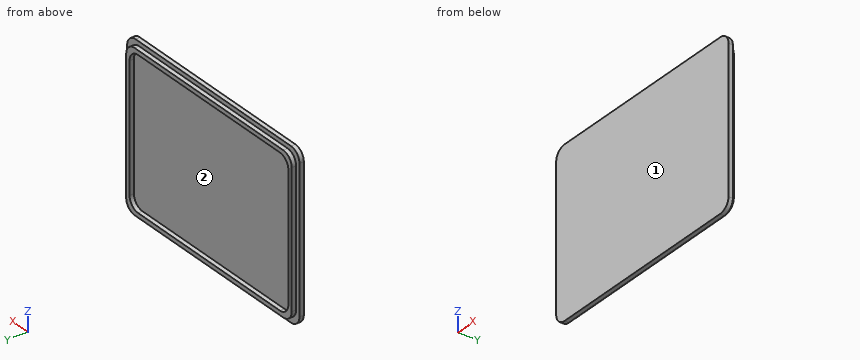
```python
from build123d import *

# Parameters (mm, degrees)
SKETCH1_W           = 101.6
SKETCH1_H           = 76.2
BOSS_EXTRUDE1_DEPTH = 2
SKETCH2_W           = 97.6
SKETCH2_H           = 72.2
SKETCH2_W_2         = 93.6
SKETCH2_H_2         = 68.2
EXTRUDE_THIN1_DEPTH = 2
FILLET1_R           = 5
FILLET2_R           = 5


with BuildPart() as part:
    # Sketch1 → Boss-Extrude1 (new body)
    with BuildSketch(Plane(origin=(0, 0, 0), x_dir=(1, 0, 0), z_dir=(0, 1, 0))):
        Rectangle(SKETCH1_W, SKETCH1_H)
    extrude(amount=BOSS_EXTRUDE1_DEPTH)

    # Sketch2 → Extrude-Thin1 (add)
    with BuildSketch(Plane(origin=(0, 2, 0), x_dir=(1, 0, 0), z_dir=(0, 1, 0))):
        Rectangle(SKETCH2_W, SKETCH2_H)
        Rectangle(SKETCH2_W_2, SKETCH2_H_2, mode=Mode.SUBTRACT)
    extrude(amount=EXTRUDE_THIN1_DEPTH)

    # Fillet1
    fillet1_edges = [part.edges().sort_by_distance(p)[0] for p in [
        (50.8, 1, 38.1),
        (-50.8, 1, 38.1),
        (-50.8, 1, -38.1),
        (50.8, 1, -38.1),
    ]]
    fillet(fillet1_edges, radius=FILLET1_R)

    # Fillet2
    fillet2_edges = [part.edges().sort_by_distance(p)[0] for p in [
        (48.8, 3, -36.1),
        (-48.8, 3, -36.1),
        (-48.8, 3, 36.1),
        (48.8, 3, 36.1),
        (-46.8, 3, -34.1),
        (-46.8, 3, 34.1),
        (46.8, 3, 34.1),
        (46.8, 3, -34.1),
    ]]
    fillet(fillet2_edges, radius=FILLET2_R)


solid = part.part
```
Verification items for the finished model (mm, model axes). Face numbers are marked on the shaded views. Round coordinates to 2 decimals unless told otherwise and drop trailing zeros. Write each loop counter-clockwise with the first axis right and the second up, starting at its lowest first coordinate (ties: lowest second). Pieces come first, ordered by that corner, then holes. Notation, with made-up numbers: (86, 7.5) - (126, 7.5) arc R17 cw to (126, 33.5) - close; hole circle Ø10 at (85, 84). An arc over 180 degrees is marked (long way). Answer as a JSON object with one key per item and string values. Group by question number.
Q1. Go/stop test with flat-tipped pins: pin 1 Ø1.5 at (x, z) = (9.5, 20.5) entering from +Y; pin 2 Ø1 at (y, z) = (3.5, 2.5) entering from -X; pin 3 Ø1 at (x, y) = (18.5, 3.5) entering from +Z. Record where each tip stops, or that it passes through.
Q2. Section check A-A, the plane y = 3.1. Enter the section's corners in (x, z), plus the area to 3 significant figures.
Q3. Mould release check, pull along Z, two halves, no side actions. Record for the marked faces 1 and 2: released by +Z, released by -Z, zero draft, split by the parting line, or undercut.
Q4. Section check B-B, the plane x = -39.5. Enter the section's corners in (y, z), plus the area to 3 significant figures.
Q5. Thickness scan on line 1 (X direction, y = 2.65, z = -19); line 2 (Z direction, x = 31.5, y = 3.2); line 3 (Y direction, x = 4.5, z = -18.5). Record the ranges inside material, lowest first.
Q6. Section check C-C, the plane z = -8.5. Enter the section's corners in (x, y).
Found:
{
 "1": {"pin 1": "stops at y = 2", "pin 2": "stops at x = -48.8", "pin 3": "stops at z = 36.1"},
 "2": {"outline": "(-48.8, -31.1) arc R5 ccw to (-43.8, -36.1) - (43.8, -36.1) arc R5 ccw to (48.8, -31.1) - (48.8, 31.1) arc R5 ccw to (43.8, 36.1) - (-43.8, 36.1) arc R5 ccw to (-48.8, 31.1) - close; hole (-46.8, -29.1) arc R5 ccw to (-41.8, -34.1) - (41.8, -34.1) arc R5 ccw to (46.8, -29.1) - (46.8, 29.1) arc R5 ccw to (41.8, 34.1) - (-41.8, 34.1) arc R5 ccw to (-46.8, 29.1) - close", "area": "663 mm^2"},
 "3": {"face 1": "zero draft", "face 2": "undercut"},
 "4": {"outline": "(0, -38.1) - (2, -38.1) - (2, -36.1) - (4, -36.1) - (4, -34.1) - (2, -34.1) - (2, 34.1) - (4, 34.1) - (4, 36.1) - (2, 36.1) - (2, 38.1) - (0, 38.1) - close", "area": "160 mm^2"},
 "5": {"line 1": "x = -48.8 to -46.8, 46.8 to 48.8", "line 2": "z = -36.1 to -34.1, 34.1 to 36.1", "line 3": "y = 0 to 2"},
 "6": {"outline": "(-50.8, 0) - (50.8, 0) - (50.8, 2) - (48.8, 2) - (48.8, 4) - (46.8, 4) - (46.8, 2) - (-46.8, 2) - (-46.8, 4) - (-48.8, 4) - (-48.8, 2) - (-50.8, 2) - close"}
}
